```python
from build123d import *

# Parameters (mm, degrees)
SKETCH1_W           = 100
SKETCH1_H           = 100
BOSS_EXTRUDE1_DEPTH = 180
SKETCH2_R           = 34.257790197
BOSS_EXTRUDE2_DEPTH = 350
SKETCH3_W           = 152.006357392
SKETCH3_H           = 282.452416457
CUT_EXTRUDE2_DEPTH  = 400
CUT_EXTRUDE3_DEPTH  = 400
CUT_EXTRUDE4_DEPTH  = 400
CUT_EXTRUDE5_DEPTH  = 400
SKETCH7_W           = 160.159381639
SKETCH7_H           = 147.362276113
CUT_EXTRUDE6_DEPTH  = 400
SKETCH8_W           = 147.310744502
SKETCH8_H           = 162.038906966
CUT_EXTRUDE7_DEPTH  = 400
SKETCH9_R           = 31.847293423
CUT_EXTRUDE8_DEPTH  = 400
SKETCH10_W          = 140.220962397
SKETCH10_H          = 212.033531124
CUT_EXTRUDE9_DEPTH  = 400


with BuildPart() as part:
    # Sketch1 → Boss-Extrude1 (new body)
    with BuildSketch(Plane(origin=(0, 0, 0), x_dir=(1, 0, 0), z_dir=(0, 1, 0))):
        with Locations((-50, 50)):
            Rectangle(SKETCH1_W, SKETCH1_H)
    extrude(amount=BOSS_EXTRUDE1_DEPTH)

    # Sketch2 → Boss-Extrude2 (add, symmetric)
    with BuildSketch(Plane(origin=(0, 180, 0), x_dir=(1, 0, 0), z_dir=(0, 1, 0))):
        with Locations(Location((-51.377291833, 49.076536384, 0), (0, 0, 270))):
            Circle(SKETCH2_R)
    extrude(amount=BOSS_EXTRUDE2_DEPTH, both=True)

    # Sketch3 → Cut-Extrude2 (cut)
    with BuildSketch(Plane(origin=(0, 0, 0), x_dir=(0, 0, -1), z_dir=(1, 0, 0))):
        with Locations((57.419900112, 502.274302507)):
            Rectangle(SKETCH3_W, SKETCH3_H)
    extrude(amount=-CUT_EXTRUDE2_DEPTH, mode=Mode.SUBTRACT)

    # Sketch4 → Cut-Extrude3 (cut)
    with BuildSketch(Plane(origin=(0, 0, 0), x_dir=(0, 0, -1), z_dir=(1, 0, 0))):
        Polygon((12.981970869, 0), (-8.994244796, 25.828096003), (-18.564506014, -15.259465835), align=None)
        Polygon((85.072517936, -1.448103984), (109.237639161, 19.113145112), (115.920034239, -3.267382694), align=None)
        Polygon((12.981970869, 180), (-8.994244796, 148.537596011), (-15.418178585, 193.219274892), align=None)
        Polygon((85.072517936, 181.854312784), (103.841225373, 159.795920888), (106.132549481, 198.647393934), align=None)
    extrude(amount=-CUT_EXTRUDE3_DEPTH, mode=Mode.SUBTRACT)

    # Sketch5 → Cut-Extrude4 (cut)
    with BuildSketch(Plane.XY):
        Polygon((-85.623287335, 0), (-106.370377984, 21.426392531), (-122.288861874, 3.209259887), (-93.526345261, -19.884701759), align=None)
        Polygon((-15.694988751, 0), (0, 15.257385304), (12.122677088, 15.257385304), (10.563067769, -19.884701759), align=None)
        Polygon((-87.166490339, 180.248071029), (-106.370377984, 151.29108453), (-117.705469457, 200.501115102), align=None)
        Polygon((-15.694988751, 180.248071029), (7.833767065, 153.279557508), (0, 193.941208308), align=None)
    extrude(amount=-CUT_EXTRUDE4_DEPTH, mode=Mode.SUBTRACT)

    # Sketch6 → Cut-Extrude5 (cut)
    with BuildSketch(Plane(origin=(0, 180, 0), x_dir=(1, 0, 0), z_dir=(0, 1, 0))):
        Polygon((-112.386997555, 28.400400964), (-64.261264503, -10.212759359), (-84.406366528, -15.51192827), (-124.649689542, -15.51192827), align=None)
        Polygon((-97.065537028, 135.861756084), (-119.37552445, 77.792688888), (-118.043343626, 64.347606737), (-66.428694172, 110.575168787), align=None)
        Polygon((-24.69640689, -21.815840769), (11.092108798, -8.97361337), (17.428316417, 32.393768119), (-38.531576846, -11.139157378), align=None)
        Polygon((-17.445484601, 140.804394854), (35.417473102, 107.262520599), (9.305452855, 72.996438725), (-31.724385352, 103.625272537), align=None)
    extrude(amount=-CUT_EXTRUDE5_DEPTH, mode=Mode.SUBTRACT)

    # Sketch7 → Cut-Extrude6 (cut)
    with BuildSketch(Plane.XY):
        with Locations((-66.123258915, -136.36252694)):
            Rectangle(SKETCH7_W, SKETCH7_H)
    extrude(amount=-CUT_EXTRUDE6_DEPTH, mode=Mode.SUBTRACT)

    # Sketch8 → Cut-Extrude7 (cut)
    with BuildSketch(Plane.XY):
        with Locations((-53.541153336, 332.448287589)):
            Rectangle(SKETCH8_W, SKETCH8_H)
    extrude(amount=-CUT_EXTRUDE7_DEPTH, mode=Mode.SUBTRACT)

    # Sketch9 → Cut-Extrude8 (cut)
    with BuildSketch(Plane(origin=(0, 251.428834106, 0), x_dir=(1, 0, 0), z_dir=(0, 1, 0))):
        with Locations(Location((-50.808993157, 49.032036374, 0), (0, 0, 270))):
            Circle(SKETCH9_R)
    extrude(amount=-CUT_EXTRUDE8_DEPTH, mode=Mode.SUBTRACT)

    # Sketch10 → Cut-Extrude9 (cut)
    with BuildSketch(Plane.ZY.offset(100)):
        with Locations((14.299084536, 180.100625535)):
            Rectangle(SKETCH10_W, SKETCH10_H)
    extrude(amount=-CUT_EXTRUDE9_DEPTH, mode=Mode.SUBTRACT)


solid = part.part
```
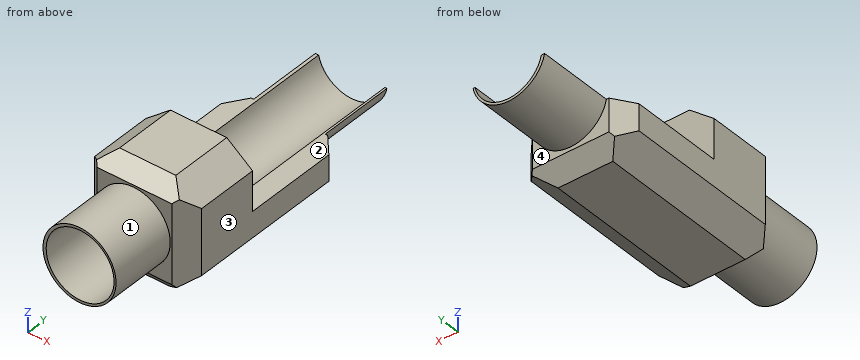
Geometry check sheet. Reference: the model listing, model coordinates, mm. Face numbers are marked on the shaded views. A direction names the side the tool comes from. Give positions to 0.01 mm unless a question says otherwise; leave off trailing zeros. Write each loop counter-clockwise with the first axis right and the second up, starting at its lowest first coordinate (ties: lowest second). Pieces come first, ordered by that corner, then holes.
1) Gauge pin test, flat ends, axial feed: pin 1 (9.5 mm diameter, centred on x = -36.5, z = -75, fed in from +Y); pin 2 (5 mm diameter, centred on y = 214.5, z = -63.5, fed in from -X); pin 3 (2 mm diameter, centred on x = -19, y = 132, fed in from -Z); pin 4 (21.5 mm diameter, centred on x = -9, y = 172, fed in from +Z). Record the tip position at first contact, or that the pin passes through.
2) Section check C-C, the plane y = 50. Record the boundary of the cut face in (x, z), and give its area (3 significant figures).
3) Access from +Z, -Z, +X, -X, +Y, -Y to the whole of each face (thin tool, end or side, straight path). Record for the marked faces 1, 2, 3 and 4.
4) Section check B-B, the plane x = -34. Record the boundary of the cut face in (y, z).
5) Material ranges on L1, parallel to Y at x = -22.5, z = -23.5; L2, parallel to Z at x = -77, y = -42; L3, parallel to X at y = 207, z = -67, recorded low to high.
6) Section check D-D, the plane y = 95. Record the boundary of the cut face in (x, z).
7) Section check A-A, the plane z = -33.5. Record the boundary of the cut face in (x, y), and give its area (3 significant figures).
Computed:
1. pin 1: stops at y = 251.43
1. pin 2: stops at x = -83.49
1. pin 3: stops at z = -94.87
1. pin 4: stops at z = -55.81
2. outline: (-100, -80.51) - (-78.24, -100) - (-26.87, -100) - (0, -79.94) - (0, -18.84) - (-24.21, 0) - (-76.99, 0) - (-100, -18.46) - close; hole circle Ø63.69 at (-50.81, -49.03)
2. area: 5,890 mm2
3. face 1: -Y
3. face 2: +Z, +X, -X, +Y
3. face 3: +Z, -Z, +X, +Y, -Y
3. face 4: -Z, +Y
4. outline: (-62.68, -78.6) - (0, -78.6) - (0, -86.77) - (11.25, -100) - (164.31, -100) - (180, -86.65) - (180, -78.6) - (251.43, -78.6) - (251.43, -76.08) - (-62.68, -76.08) - close; (-62.68, -21.98) - (74.08, -21.98) - (74.08, 0) - (15.26, 0) - (0, -12.98) - (0, -19.55) - (-62.68, -19.55) - close
5. L1: y = 0 to 74.08
5. L2: z = -71.82 to -67.15, -30.91 to -26.34
5. L3: x = -80.57 to -77.1, -24.51 to -22.18
6. outline: (-100, -80.51) - (-78.24, -100) - (-26.87, -100) - (0, -79.94) - (0, -55.81) - (-19.69, -55.81) arc R31.85 cw to (-81.93, -55.81) - (-100, -55.81) - close
7. outline: (-100, 14.85) - (-85.62, 0) - (-81.89, 0) - (-81.89, -62.68) - (-78.61, -62.68) - (-78.61, 74.08) - (-100, 74.08) - close; (-23.01, -62.68) - (-20.87, -62.68) - (-20.87, 0) - (-15.69, 0) - (0, 15.26) - (0, 74.08) - (-23.01, 74.08) - close
7. area: 3,400 mm2
